```python
from build123d import *

# Parameters (mm, degrees)
CYLINDER_R     = 2
CYLINDER_DEPTH = 12
EXTRUDE_DEPTH  = 10


with BuildPart() as cilindro:
    # Cylinder → Cylinder (new body)
    with BuildSketch(Plane(origin=(59.98, -74.8, 0), x_dir=(1, 0, 0), z_dir=(0, 0, 1))):
        Circle(CYLINDER_R)
    extrude(amount=CYLINDER_DEPTH)


with BuildPart() as cut:
    # path2246 → Extrude (new body)
    with BuildSketch(Plane(origin=(94.341844, -105.754461, 0), x_dir=(0, -1, 0), z_dir=(0, 0, -1))):
        with BuildLine():
            add(Edge.make_bspline(
                [(41.622189, 0.139513), (-3.420731, 40.581559)],
                knots=[0, 0, 60.534484, 60.534484], degree=1))
            add(Edge.make_bspline(
                [(-3.420731, 40.581559), (-3.420731, 40.581559), (-24.478139, 55.667165), (-33.827718, 36.291336)],
                knots=[0, 0, 0, 0, 1, 1, 1, 1], degree=3))
            add(Edge.make_bspline(
                [(-33.827718, 36.291336), (-46.948673, 9.099806), (-15.449255, 2.542274), (-15.449255, 2.542274)],
                knots=[0, 0, 0, 0, 1, 1, 1, 1], degree=3))
            add(Edge.make_bspline(
                [(-15.449255, 2.542274), (-15.449255, 2.542274), (-34.638948, -15.120666), (-34.659558, -24.840656)],
                knots=[0, 0, 0, 0, 1, 1, 1, 1], degree=3))
            add(Edge.make_bspline(
                [(-34.659558, -24.840656), (-35.31742, -50.902936), (-1.036181, -48.507456), (4.117339, -36.979596)],
                knots=[0, 0, 0, 0, 1, 1, 1, 1], degree=3))
            add(Edge.make_bspline(
                [(4.117339, -36.979596), (13.587039, -28.871746), (41.622189, 0.139513), (41.622189, 0.139513)],
                knots=[0, 0, 0, 0, 1, 1, 1, 1], degree=3))
        make_face()
    extrude(amount=-EXTRUDE_DEPTH)

    # Cut: cut Cilindro
    add(cilindro.part, mode=Mode.SUBTRACT)


solid = cut.part
```
Here's how the part is built. I have some questions about the finished solid (model axes, mm). Coordinates: 2 decimals unless noted, no trailing zeros.
1) We'd pull the mould along X, two halves only. Please class faces 1 (the face through (91, -102, 10)), 2 (the face through (59.72, -72.817, 4.93)): +X half, -X half, draft (parallel to the pull), parting line (faces both ways), or undercut.
2) Will these pins go through, and if not, where does the flat tip stop? pin 1 (4 mm diameter, centred on x = 62.5, z = 5.5, fed in from +Y); pin 2 (6 mm diameter, centred on y = -126.5, z = 3, fed in from +X); pin 3 (5 mm diameter, centred on x = 111.5, z = 7, fed in from -Y).
3) I need wall thicknesses on line 1 (X direction, y = -74.8, z = 2.5); line 2 (Y direction, x = 59.98, z = 4.25); line 3 (X direction, y = -87, z = 2.5). Which ranges of each line are inside material? Lowest first, please.
4) Imagine slicing it at A-A on y = -74.8. State how many separate pieces and enclosed holes the cut face has, and give its area (3 significant figures).
Response values:
1. face 1: draft
1. face 2: undercut
2. pin 1: stops at y = -69.51
2. pin 2: stops at x = 118.4
2. pin 3: stops at y = -132.89
3. line 1: x = 53.51 to 57.98, 61.98 to 83.91, 109.68 to 132.14
3. line 2: y = -109.26 to -76.8, -72.8 to -71.06
3. line 3: x = 48.18 to 90.86, 95.02 to 139.14
4. separate pieces: 3
4. enclosed holes: 0
4. area: 489 mm2
